from build123d import *

# Parameters (mm, degrees)
CUT_EXTRUDE1_DEPTH      = 71.032135481
CUT_EXTRUDE1_DEPTH_BACK = 71.032135481
SKETCH2_R               = 1
CHAMFER1_SIZE           = 0.2
CUT_EXTRUDE2_DEPTH      = 71.032135485
CUT_EXTRUDE2_DEPTH_BACK = 71.032135485
SKETCH3_W               = 9
SKETCH3_H               = 1


with BuildPart() as part:
    # Sketch1 → Revolve1 (revolve)
    with BuildSketch(Plane.XY):
        Polygon((-70, 0), (-70, 1.5), (0, 1.5), (0, 0.5), (0, 0), (-9, 0), align=None)
    revolve(axis=Axis((0, 0, 0), (-1, 0, 0)))

    # Sketch2 → Cut-Extrude1 (cut, two sides: drawn at the far end of the back side and taken through both)
    with BuildSketch(Plane.XY.offset(-CUT_EXTRUDE1_DEPTH_BACK)):
        with Locations((-3, 0)):
            Circle(SKETCH2_R)
    extrude(amount=CUT_EXTRUDE1_DEPTH + CUT_EXTRUDE1_DEPTH_BACK, mode=Mode.SUBTRACT)

    # Chamfer1
    chamfer1_edges = [part.edges().sort_by_distance(p)[0] for p in [
        (0, -1.5, 0),
        (-70, -1.5, 0),
    ]]
    chamfer(chamfer1_edges, length=CHAMFER1_SIZE)

    # Sketch3 → Cut-Extrude2 (cut, two sides: drawn at the far end of the back side and taken through both)
    with BuildSketch(Plane(origin=(0, 0, 0), x_dir=(1, 0, 0), z_dir=(0, 1, 0)).offset(-CUT_EXTRUDE2_DEPTH_BACK)):
        with Locations((-4.5, 0)):
            Rectangle(SKETCH3_W, SKETCH3_H)
    extrude(amount=CUT_EXTRUDE2_DEPTH + CUT_EXTRUDE2_DEPTH_BACK, mode=Mode.SUBTRACT)


solid = part.part
Verification items for the finished model (mm, model axes). Round coordinates to 2 decimals unless told otherwise and drop trailing zeros. Loops run counter-clockwise (first coordinate to the right, second up) from the corner with the lowest first, then second, coordinate; pieces in that order, holes last. Notation, with made-up numbers: (26, 74.5) - (71, 74.5) arc R20 ccw to (71, 89.5) - close; hole circle Ø6 at (14.25, 39). An arc over 180 degrees is marked (long way). Answer in a Markdown table with one row per item. Add a question column.
Q1. Gauge pin test, flat end, axial feed: pin 1 (0.8 mm diameter, centred on y = -0.5, z = 0, fed in from +X). Record the tip position at first contact, or that the pin passes through.
Q2. Release check for a two-part mould opening along Z. For faces 1 (the face through (-70, 0, 0)), 2 (the face through (-34.5, -1.2, 0.9)), 3 (the face through (-5, 0, -0.5)), 4 (the face through (-5, 0, 0.5)) record: pulls with the +Z half, pulls with the -Z half, needs draft (parallel to the pull), parting line crosses it, or undercut.
Q3. Section check D-D on x = -53.5. Enter the section's corners in (y, z), plus the area to 3 significant figures.
Q4. Section check C-C on z = 0. Enter the section's corners in (x, y).
Q5. Section check B-B on x = -3. Enter the section's corners in (y, z).
Q6. Material ranges on line 1 (X direction, y = 0, z = 0.8); line 2 (Y direction, x = -3, z = 0.9); line 3 (X direction, y = 0.8, z = 0.4), recorded low to high.
Q7. Section check A-A on y = 0. Enter the section's corners in (x, z), plus the area to 3 significant figures.
Found:
| question | item | result |
|---|---|---|
| 1 | pin 1 | stops at x = -9 |
| 2 | face 1 | needs draft |
| 2 | face 2 | parting line crosses it |
| 2 | face 3 | undercut |
| 2 | face 4 | undercut |
| 3 | outline | circle Ø3 at (0, 0) |
| 3 | area | 7.07 mm² |
| 4 | outline | (-70, -1.3) - (-69.8, -1.5) - (-9, -1.5) - (-9, 1.5) - (-69.8, 1.5) - (-70, 1.3) - close |
| 5 | outline | (-1.41, -0.5) arc R1.5 ccw to (-1, -1.12) - (-1, -0.5) - close; (-1.41, 0.5) - (-1, 0.5) - (-1, 1.12) arc R1.5 ccw to start; (1, -1.12) arc R1.5 ccw to (1.41, -0.5) - (1, -0.5) - close; (1, 0.5) - (1.41, 0.5) arc R1.5 ccw to (1, 1.12) - close |
| 6 | line 1 | x = -70 to -4, -2 to 0 |
| 6 | line 2 | y = -1.2 to -1, 1 to 1.2 |
| 6 | line 3 | x = -70 to -9 |
| 7 | outline | (-70, -1.3) - (-69.8, -1.5) - (-4, -1.5) - (-4, -0.5) - (-9, -0.5) - (-9, 0.5) - (-4, 0.5) - (-4, 1.5) - (-69.8, 1.5) - (-70, 1.3) - close; (-2, -1.5) - (-0.2, -1.5) - (0, -1.3) - (0, -0.5) - (-2, -0.5) - close; (-2, 0.5) - (0, 0.5) - (0, 1.3) - (-0.2, 1.5) - (-2, 1.5) - close |
| 7 | area | 197 mm² |
